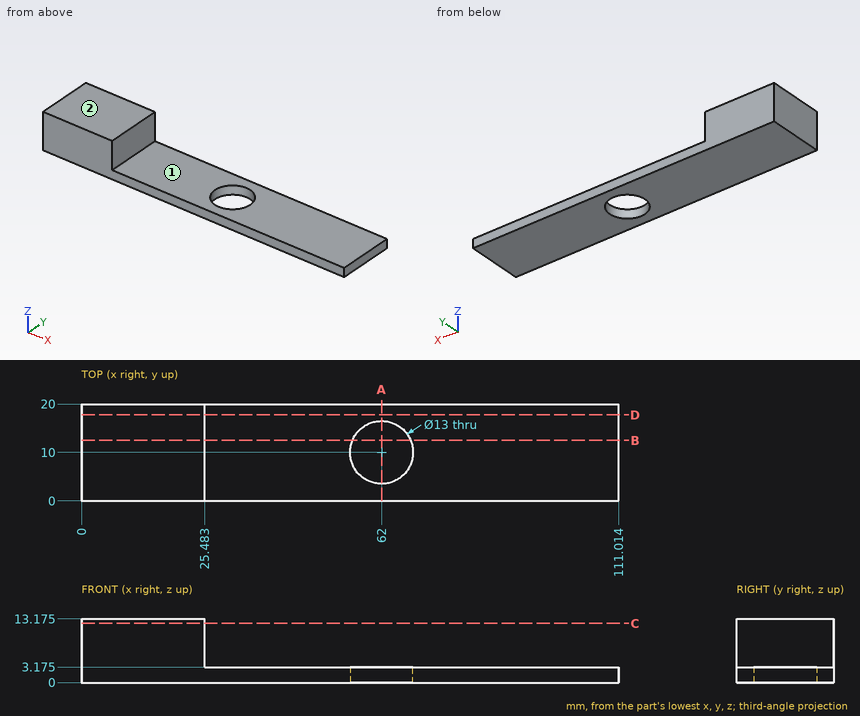
For this review, use the dimensioned drawing (mm, ordinates from the lowest corner) and the shaded views. A direction names the side the tool comes from. Give positions to 0.01 mm unless a question says otherwise; leave off trailing zeros. Write each loop counter-clockwise with the first axis right and the second up, starting at its lowest first coordinate (ties: lowest second). Pieces come first, ordered by that corner, then holes. Notation, with made-up numbers: M -29.5,7 L 18.5,7 A13 cw 18.5,22 Z; hole C -39,-31 d1. An arc over 180 degrees is marked long. Write item = value, one per line. Start each with the question number.
Q1. Clearance check with flat-ended pins moving along their axes: pin 1 (10.5 mm diameter, centred on x = 62, y = 10, fed in from -Z); pin 2 (8 mm diameter, centred on x = 90, y = 15, fed in from +Z) (3 decimals); pin 3 (2 mm diameter, centred on y = 17, z = 9.5, fed in from +X). State where each tip first meets the part, or that it passes through.
Q2. We need section C-C (z = 12.25). State the section outline as (x, y) points, plus the area to 3 significant figures.
Q3. We need section D-D (y = 17.75). State the section outline as (x, z) points (1 decimal).
Q4. For line 1 (Y direction, x = 62, z = 1.5); line 2 (X direction, y = 10, z = 1.4); line 3 (X direction, y = 6.75, z = 8.5), list the stretches that pass through material, from the lowest coordinate up.
Q5. Machinability: for the marked faces 1 and 2, which of the approach directions +Z, -Z, +X, -X, +Y, -Y give a long, thin tool a straight path to every point of the face, cutting with its end or side? Answer none if there is none.
Q6. We need section B-B (y = 12.5). State the section outline as (x, z) points (1 decimal), plus the area to 3 significant figures.
Q7. We need section A-A (x = 62). State the section outline as (y, z) points (1 decimal), plus the area to 3 significant figures.
Result set:
q1.pin_1 = through
q1.pin_2 = 3.175
q1.pin_3 = 25.48
q2.outline = M 0,0 L 25.48,0 L 25.48,20 L 0,20 Z
q2.area = 510 mm2
q3.outline = M 0,0 L 111,0 L 111,3.2 L 25.5,3.2 L 25.5,13.2 L 0,13.2 Z
q4.line_1 = 0 to 3.5, 16.5 to 20
q4.line_2 = 0 to 55.5, 68.5 to 111.01
q4.line_3 = 0 to 25.48
q5.face_1 = +Z, +X, +Y, -Y
q5.face_2 = +Z, +X, -X, +Y, -Y
q6.outline = M 0,0 L 56,0 L 56,3.2 L 25.5,3.2 L 25.5,13.2 L 0,13.2 Z; M 68,0 L 111,0 L 111,3.2 L 68,3.2 Z
q6.area = 569 mm2
q7.outline = M 0,0 L 3.5,0 L 3.5,3.2 L 0,3.2 Z; M 16.5,0 L 20,0 L 20,3.2 L 16.5,3.2 Z
q7.area = 22.2 mm2
